Model file for the job. Use its own axes, mm. Give positions to 0.01 mm unless a question says otherwise; leave off trailing zeros. Order: outer loops, then holes, each group sorted by start corner. A loop starts at its lowest first (then second) coordinate and runs counter-clockwise, first axis right, second up. Notation, with made-up numbers: (54.25, 50) - (64.25, 50) arc R22 cw to (64.25, 71) - close; hole circle Ø9 at (-24.75, 39). An arc over 180 degrees is marked (long way). Use CSV: the item, a comma, the result in double quotes. Start each with the question number.
(1) Probe L1, parallel to X at y = -36.5, z = 0.6; L2, parallel to Y at x = 50, z = 2.15; L3, parallel to X at y = 49.5, z = 1.95. List the from-to ranges inside material, lowest first.
(2) Drop flat-ended pins along their axis: pin 1 Ø1 at (y, z) = (-54, 2.5) entering from -X; pin 2 Ø1 at (y, z) = (54.5, 1) entering from +X. Give the stop position or say it passes through.
(3) Pull direction X, two halves, no side cores. Call faces 1 (the cylindrical face through (62.31, 59.04, 1.48)), 2 (the flat face through (-1, 19, 3)), 3 (the cylindrical face through (52.31, 59.04, 1.48)): +X half, -X half, draft (parallel to the pull), parting line (faces both ways), or undercut.
(4) Band-saw the part on B-B, the plane y = -65. Give the cut face in (x, z), then the cut area to 3 significant figures.
(5) Band-saw the part on A-A, the plane x = 60. Give the cut face in (y, z).
(6) Band-saw the part on C-C, the plane z = 2.35. Count the separate pieces of the cut face and the enclosed holes in it, then the cut area to 3 significant figures.
from build123d import *

# Parameters (mm, degrees)
SKETCH1_W           = 17
SKETCH1_H           = 16
SKETCH1_R           = 2.5
BOSS_EXTRUDE1_DEPTH = 3
SKETCH2_W           = 3
SKETCH2_H           = 40
CUT_EXTRUDE1_DEPTH  = 114.176852757


with BuildPart() as part:
    # Sketch1 → Boss-Extrude1 (new body)
    with BuildSketch(Plane.XY):
        Polygon((80, 80), (-80, 80), (-80, -80), (-25, -80), (-25, 10), (25, 10), (25, -80), (80, -80), align=None)
        with Locations((0, 52)):
            Rectangle(SKETCH1_W, SKETCH1_H, mode=Mode.SUBTRACT)
        with Locations((50, 60)):
            Circle(SKETCH1_R, mode=Mode.SUBTRACT)
        with Locations((60, 60)):
            Circle(SKETCH1_R, mode=Mode.SUBTRACT)
    extrude(amount=BOSS_EXTRUDE1_DEPTH)

    # Sketch2 → Cut-Extrude1 (cut, through all)
    with BuildSketch(Plane.XY.offset(3)):
        with Locations((-78.5, 40)):
            Rectangle(SKETCH2_W, SKETCH2_H)
        with Locations((-78.5, -40)):
            Rectangle(SKETCH2_W, SKETCH2_H)
        with Locations((78.5, -40)):
            Rectangle(SKETCH2_W, SKETCH2_H)
        with Locations((78.5, 40)):
            Rectangle(SKETCH2_W, SKETCH2_H)
    extrude(amount=-CUT_EXTRUDE1_DEPTH, mode=Mode.SUBTRACT)


solid = part.part
Answer block:
1,L1,"x = -77 to -25, 25 to 77"
1,L2,"y = -80 to 57.5, 62.5 to 80"
1,L3,"x = -77 to -8.5, 8.5 to 77"
2,pin 1,"stops at x = -77"
2,pin 2,"stops at x = 77"
3,face 1,"undercut"
3,face 2,"draft"
3,face 3,"undercut"
4,outline,"(-80, 0) - (-25, 0) - (-25, 3) - (-80, 3) - close; (25, 0) - (80, 0) - (80, 3) - (25, 3) - close"
4,area,"330 mm2"
5,outline,"(-80, 0) - (57.5, 0) - (57.5, 3) - (-80, 3) - close; (62.5, 0) - (80, 0) - (80, 3) - (62.5, 3) - close"
6,separate pieces,"1"
6,enclosed holes,"3"
6,area,"20,300 mm2"
